Source: three-view drawing plus pictorial views. Frame: mm from the lowest corner of the part. A direction names the side the tool comes from. Coordinates: 2 decimals unless noted, no trailing zeros. Write each loop counter-clockwise with the first axis right and the second up, starting at its lowest first coordinate (ties: lowest second). Pieces come first, ordered by that corner, then holes. Notation, with made-up numbers: (65, 50.5) -> (99, 50.5) arc R16 cw to (99, 81.5) -> close; hole circle Ø6 at (-35, -32.5). An arc over 180 degrees is marked (long way). One line per item, written item: value.
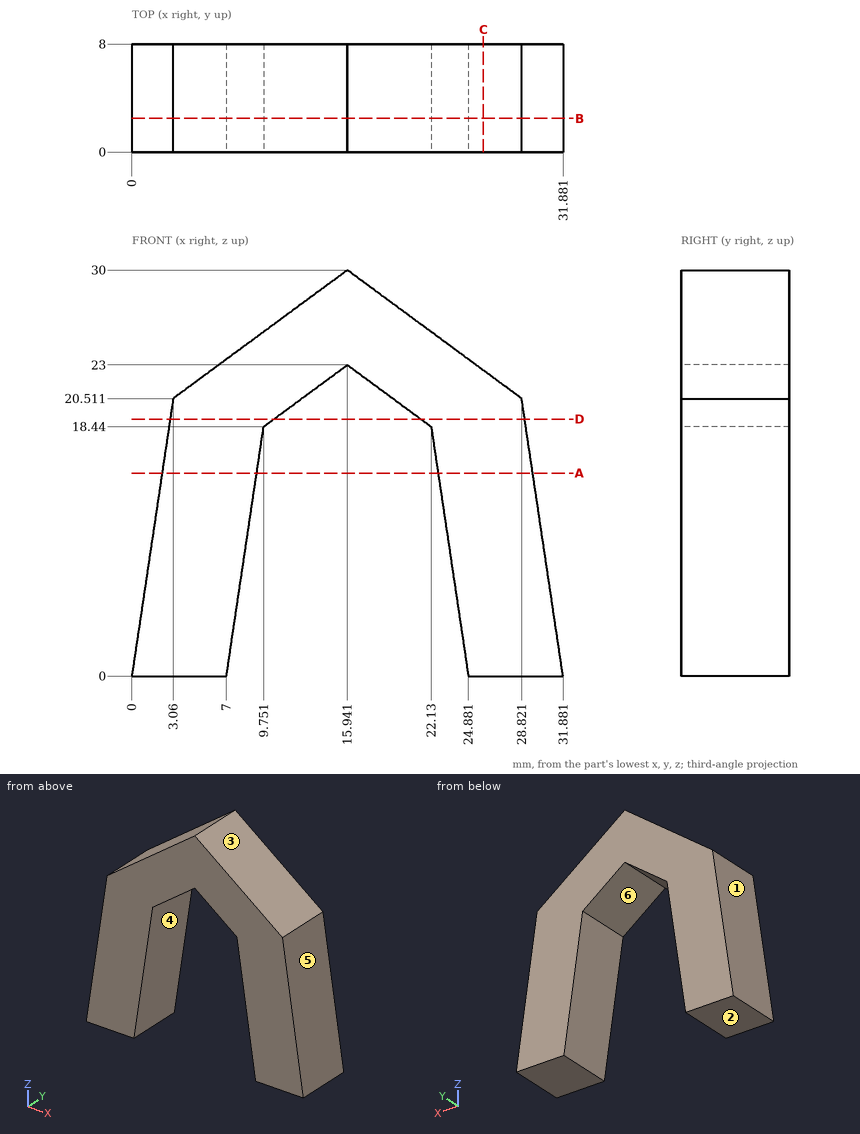
(1) Section C-C (x = 26). Return the cut outline in (y, z), then the cut area to 3 significant figures.
Responses:
outline: (0, 0) -> (8, 0) -> (8, 22.59) -> (0, 22.59) -> close
area: 181 mm2
(2) Section B-B (y = 2.5). Return the cut outline in (x, z).
Responses:
outline: (0, 0) -> (7, 0) -> (9.75, 18.44) -> (15.94, 23) -> (22.13, 18.44) -> (24.88, 0) -> (31.88, 0) -> (28.82, 20.51) -> (15.94, 30) -> (3.06, 20.51) -> close
(3) First-contact query: pin 1 (1 mm diameter, centred on x = 17, y = 5, fed in from +Z); pin 2 (2 mm diameter, centred on x = 12.5, y = 4, fed in from -Z); pin 3 (2 mm diameter, centred on y = 5.5, z = 25.5, fed in from +X) (1 decimal). Flat tips, straight axial feed; report the tip coordinate or a pass-through.
Responses:
pin 1: stops at z = 29.59
pin 2: stops at z = 19.73
pin 3: stops at x = 23.4
(4) Section D-D (z = 19). Return the cut outline in (x, y) (1 decimal), then the cut area to 3 significant figures.
Responses:
outline: (2.8, 0) -> (10.5, 0) -> (10.5, 8) -> (2.8, 8) -> close; (21.4, 0) -> (29, 0) -> (29, 8) -> (21.4, 8) -> close
area: 123 mm2
(5) Line query: line 1 (X direction, y = 3, z = 12); line 2 (X direction, y = 7.5, z = 4.5); line 3 (Z direction, x = 26, y = 6.75). Output: solid intervals per line, ascending. Write a range as [from, to].
Responses:
line 1: x = [1.79, 8.79], [23.09, 30.09]
line 2: x = [0.67, 7.67], [24.21, 31.21]
line 3: z = [0, 22.59]
(6) Section A-A (z = 15). Return the cut outline in (x, y).
Responses:
outline: (2.24, 0) -> (9.24, 0) -> (9.24, 8) -> (2.24, 8) -> close; (22.64, 0) -> (29.64, 0) -> (29.64, 8) -> (22.64, 8) -> close
(7) Pull-direction query (X, two-part tool) for the marked faces 1, 2, 3 and 4; classes: released by +X, released by -X, zero draft, split by the parting line, or undercut.
Responses:
face 1: released by -X
face 2: zero draft
face 3: released by +X
face 4: undercut
(8) Reachability of the marked faces 5 and 6 from +Z, -Z, +X, -X, +Y, -Y: full face, straight path, thin tool, end or side. Return the list, or none.
Responses:
face 5: +Z, +X, +Y, -Y
face 6: -Z, +Y, -Y
